Can you work these out from the model? Positions are in its coordinate system, mm. Face numbers are marked on the shaded views. A direction names the side the tool comes from. Give positions to 0.01 mm unless a question says otherwise; leave off trailing zeros. Loops run counter-clockwise (first coordinate to the right, second up) from the corner with the lowest first, then second, coordinate; pieces in that order, holes last. Notation, with made-up numbers: M 36.5,-25.75 L 42.5,-25.75 A12 ccw 42.5,-11.75 Z; hole C 22,6.25 d2. An arc over 180 degrees is marked long. Use CSV: the item, a comma, the result in double quotes.
from build123d import *

# Parameters (mm, degrees)
SKETCH_1_W      = 90
SKETCH_1_H      = 90
EXTRUDE_1_DEPTH = 2
EXTRUDE_5_DEPTH = 9


with BuildPart() as part:
    # 草图1 → 凸台-拉伸1 (new body)
    with BuildSketch(Plane(origin=(0, 0, 0), x_dir=(1, 0, 0), z_dir=(0, 1, 0))):
        Rectangle(SKETCH_1_W, SKETCH_1_H)
    extrude(amount=EXTRUDE_1_DEPTH)

    # 草图2 → 拉伸-薄壁5 (add)
    with BuildSketch(Plane(origin=(0, 2, 0), x_dir=(1, 0, 0), z_dir=(0, 1, 0))):
        with BuildLine():
            Line((40.343110101, -45), (40.343110101, -32.015885558))
            ThreePointArc((40.343110101, -32.015885558), (19.254798346, 18.895802688), (-31.656889899, 39.984114442))
            Line((-31.656889899, 39.984114442), (-45, 39.984114442))
            Line((-45, 39.984114442), (-45, 37.984114442))
            Line((-45, 37.984114442), (-31.656889899, 37.984114442))
            ThreePointArc((-31.656889899, 37.984114442), (17.840584784, 17.481589125), (38.343110101, -32.015885558))
            Line((38.343110101, -32.015885558), (38.343110101, -45))
            Line((38.343110101, -45), (40.343110101, -45))
        make_face()
        with BuildLine():
            Line((28.343110101, -45), (28.343110101, -32.015885558))
            ThreePointArc((28.343110101, -32.015885558), (10.769516972, 10.410521313), (-31.656889899, 27.984114442))
            Line((-31.656889899, 27.984114442), (-45, 27.984114442))
            Line((-45, 27.984114442), (-45, 25.984114442))
            Line((-45, 25.984114442), (-31.656889899, 25.984114442))
            ThreePointArc((-31.656889899, 25.984114442), (9.35530341, 8.996307751), (26.343110101, -32.015885558))
            Line((26.343110101, -32.015885558), (26.343110101, -45))
            Line((26.343110101, -45), (28.343110101, -45))
        make_face()
    extrude(amount=EXTRUDE_5_DEPTH)


solid = part.part
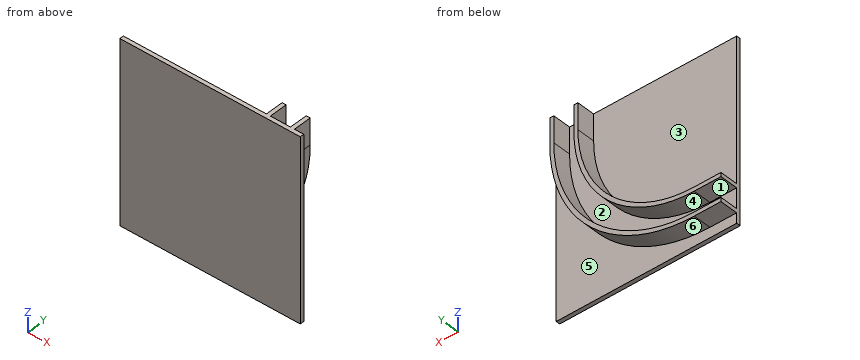
Q1. For the marked faces 1, 2 and 3, which set-ups out of +Z, -Z, +X, -X, +Y, -Y let a thin tool reach every point of the face, with its end or its side?
Model answer:
face 1,"-X, +Y"
face 2,"+Y"
face 3,"+Z, -X, +Y"
Q2. I want a section at B-B, the plane x = 33.5. Please give me the cut outline in (y, z), then the cut area to 3 significant figures.
Model answer:
outline,"M 0,-45 L 2,-45 L 2,1.38 L 11,1.38 L 11,6.43 L 2,6.43 L 2,45 L 0,45 Z"
area,"225 mm2"
Q3. I want a section at D-D, the plane x = -34. Please give me the cut outline in (y, z), then the cut area to 3 significant figures.
Model answer:
outline,"M 0,-45 L 2,-45 L 2,-39.98 L 11,-39.98 L 11,-37.98 L 2,-37.98 L 2,-27.98 L 11,-27.98 L 11,-25.98 L 2,-25.98 L 2,45 L 0,45 Z"
area,"216 mm2"
Q4. I'm going to push flat-ended pins straight in: P1, Ø6, axis at x = 25.5, y = 3.5, coming from the +Z side; P2, Ø5, axis at x = -29.5, z = 22.5, coming from the +Y side; P3, Ø2, axis at x = -29, y = 4, coming from the +Z side; P4, Ø4.5, axis at x = -37.5, y = 7.5, coming from the +Z side. Where does each tip first touch, or does it pass through?
Model answer:
P1,"z = 45"
P2,"y = 2"
P3,"z = -25.87"
P4,"z = -25.98"
Q5. I want a section at C-C, the plane z = 16. Please give me the cut outline in (x, y).
Model answer:
outline,"M -45,0 L 45,0 L 45,2 L 38.54,2 L 38.54,11 L 36.49,11 L 36.49,2 L 26.17,2 L 26.17,11 L 24.09,11 L 24.09,2 L -45,2 Z"
Q6. Please list where these lines run through material, in increasing order: L1, parallel to X at y = 10, z = 38.5; L2, parallel to Y at x = -8, z = 26; L3, parallel to X at y = 4, z = -11. Write a range as from..to.
Model answer:
L1,"26.34..28.34, 38.34..40.34"
L2,"0..2"
L3,"7.25..10.17, 23.57..26.08"
Q7. If we mould it in two halves opening along Z, with no side actions, what happens to the marked faces 4, 5 and 6? For each: released by +Z, released by -Z, zero draft, split by the parting line, or undercut.
Model answer:
face 4,"undercut"
face 5,"zero draft"
face 6,"released by -Z"
Q8. I want a section at A-A, the plane y = 3.25. Please give me the cut outline in (x, z), then the cut area to 3 significant figures.
Model answer:
outline,"M -45,-39.98 L -31.66,-39.98 A72 ccw 40.34,32.02 L 40.34,45 L 38.34,45 L 38.34,32.02 A70 cw -31.66,-37.98 L -45,-37.98 Z; M -45,-27.98 L -31.66,-27.98 A60 ccw 28.34,32.02 L 28.34,45 L 26.34,45 L 26.34,32.02 A58 cw -31.66,-25.98 L -45,-25.98 Z"
area,"514 mm2"
